Design review of the part built by this model. Coordinates are the model's own, in mm. A direction names the side the tool comes from. Round coordinates to 2 decimals unless told otherwise and drop trailing zeros. Write each loop counter-clockwise with the first axis right and the second up, starting at its lowest first coordinate (ties: lowest second). Pieces come first, ordered by that corner, then holes. Notation, with made-up numbers: (17, -27.5) -> (74, -27.5) arc R13 cw to (74, -7.5) -> close; hole circle Ø6 at (5.5, 6.25). An arc over 180 degrees is marked (long way). Write item = value, one per line. Start each with the question number.
Item 1: Add section D-D, the plane z = 12. State the section outline as (x, y) points, then the cut area to 3 significant figures.
Item 2: Machinability: for faces 1 (the cylindrical face through (20.8, 31.08, -2.11)), 2 (the cylindrical face through (12, 33, 0)), which of the approach directions +Z, -Z, +X, -X, +Y, -Y give a long, thin tool a straight path to every point of the face, cutting with its end or side? Answer none if there is none.
Item 3: Add section B-B, the plane x = 8. State the section outline as (y, z) points, then the cut area to 3 significant figures.
Item 4: To check wall thickness, follow L1, parallel to X at y = 0, z = -17.5; L2, parallel to X at y = 0, z = -16; L3, parallel to Y at x = 1.5, z = -0.5. State the ranges of each line that lie inside material, in increasing order.
Item 5: For pin 1 Ø23.5 at (y, z) = (0, 0) entering from +X; pin 2 Ø8.5 at (y, z) = (26, 0) entering from +X; pin 3 Ø5.5 at (y, z) = (25, 0.5) entering from +X; pin 4 Ø12 at (x, z) = (13.5, -1.5) entering from +Y, all flat-tipped, find the tip position at first contact; note any pin that passes through.
Item 6: Add section A-A, the plane y = 0. State the section outline as (x, z) points.
Item 7: Add section C-C, the plane x = 19.75. State the section outline as (y, z) points, then the cut area to 3 significant figures.
Item 8: Mouldability with a two-part tool opening along Z and no side actions: class faces 3 (the flat face through (24, -8, 15)), 4 (the cylindrical face through (8.86, 23.36, -2.02)), 5 (the cylindrical face through (12, -33, 0)) as released by +Z, released by -Z, zero draft, split by the parting line, or undercut.
Autodesk Inventor part; units mm, degrees
ref_plane "to_bearings_XY" through (16, 0, 0) normal (1, 0, 0) x (0, 0, -1)
ref_plane "to_bearings_YZ" through (16, 0, 0) normal (0, 0, -1) x (0, 1, 0)
ref_plane "to_bearings_ZX" through (16, 0, 0) normal (0, 1, 0) x (1, 0, 0)
sketch "Sketch_1" plane through (0, 0, 0) normal (0, 0, 1) x (1, 0, 0)
  line L0 (24, 0) -> (0, 0)
  line L1 (0, 33) -> (0, 13)
  line L2 (0, 13) -> (16, 13)
  line L3 (16, 13) -> (16, 16.5)
  line L4 (16, 16.5) -> (24, 16.5)
  line L5 (24, 16.5) -> (24, 33)
  line L6 (24, 33) -> (0, 33)
revolve "Revolution1" add sketch "Sketch_1" angle 360 about axis through (24, 0, 0) along (1, 0, 0)
sketch "Sketch_2" plane through (0, 0, 0) normal (1, 0, 0) x (0, 1, 0)
  line L0 (-132, 88) -> (-132, -88)
  line L1 (-132, -88) -> (132, -88)
  line L2 (132, -88) -> (132, 88)
  line L3 (132, 88) -> (-132, 88)
  line L4 (-33, 22) -> (-33, -22)
  line L5 (-33, -22) -> (33, -22)
  line L6 (33, -22) -> (33, 22)
  line L7 (33, 22) -> (-33, 22)
extrude "Extrusion1" cut sketch "Sketch_2" along normal blind 26
sketch "Sketch_3" plane through (0, 0, 0) normal (0, 0, 1) x (1, 0, 0)
  line L0 (24, 26) -> (0, 26)
  line L1 (0, 26) -> (0, 30)
  line L2 (0, 30) -> (0.6765, 29.3235)
  line L3 (0.6765, 29.3235) -> (16.8235, 29.3235)
  line L4 (16.8235, 29.3235) -> (17.5, 30)
  line L5 (17.5, 30) -> (17.5, 31.5)
  line L6 (17.5, 31.5) -> (24, 31.5)
  line L7 (24, 31.5) -> (24, 26)
  line L8 (24, 26) -> (0, 26)
revolve "Revolution2" cut sketch "Sketch_3" angle 360 about axis through (24, 26, 0) along (1, 0, 0)
thread "Thread1"
pattern_linear "Rectangular Pattern1" count 2 spacing 52 along (0, -1, 0) of "Revolution2"
sketch "Sketch_4" plane through (8, 0, 0) normal (1, 0, 0) x (0, 0, -1)
  line L0 (-12.65, 0) -> (-22, 0)
  line L1 (-22, 0) -> (-22, 2.5)
  line L2 (-22, 2.5) -> (-21.567, 2.067)
  line L3 (-21.567, 2.067) -> (-13.083, 2.067)
  line L4 (-13.083, 2.067) -> (-12.65, 2.5)
  line L5 (-12.65, 2.5) -> (-12.65, 0)
  line L6 (-12.65, 0) -> (-22, 0)
revolve "Revolution3" cut sketch "Sketch_4" angle 360 about axis through (8, 0, 12.65) along (0, 0, -1)
thread "Thread2"
sketch "Sketch_6" plane through (8, 0, 0) normal (1, 0, 0) x (0, 0, -1)
  line L0 (22, 0) -> (12.65, 0)
  line L1 (12.65, 0) -> (12.65, 2.5)
  line L2 (12.65, 2.5) -> (13.083, 2.067)
  line L3 (13.083, 2.067) -> (21.567, 2.067)
  line L4 (21.567, 2.067) -> (22, 2.5)
  line L5 (22, 2.5) -> (22, 0)
  line L6 (22, 0) -> (12.65, 0)
revolve "Revolution4" cut sketch "Sketch_6" angle 360 about axis through (8, 0, -22) along (0, 0, -1)
thread "Thread3"
ref_plane "to_bearings_XY" through (16, 0, 0) normal (1, 0, 0) x (0, 0, -1)
ref_plane "to_bearings_YZ" through (16, 0, 0) normal (0, 0, -1) x (0, 1, 0)
ref_plane "to_bearings_ZX" through (16, 0, 0) normal (0, 1, 0) x (1, 0, 0)
ref_plane "to_screw1_XY" through (8, 0, 13) normal (0, 0, 1) x (1, 0, 0)
ref_plane "to_screw1_YZ" through (8, 0, 13) normal (1, 0, 0) x (0, 1, 0)
ref_plane "to_screw1_ZX" through (8, 0, 13) normal (0, 1, 0) x (0, 0, 1)
ref_plane "to_screw2_XY" through (8, 0, -13) normal (0, 0, -1) x (1, 0, 0)
ref_plane "to_screw2_YZ" through (8, 0, -13) normal (1, 0, 0) x (0, -1, 0)
ref_plane "to_screw2_ZX" through (8, 0, -13) normal (0, -1, 0) x (0, 0, -1)
properties part number "BGCSB14_h"
Result set:
q1.outline = (0, -30.74) -> (24, -30.74) -> (24, -11.32) -> (16, -11.32) -> (16, -5) -> (0, -5) -> close; (0, 5) -> (16, 5) -> (16, 11.32) -> (24, 11.32) -> (24, 30.74) -> (0, 30.74) -> close
q1.area = 1,130 mm²
q2.face_1 = +X
q2.face_2 = +X, -X, +Y
q3.outline = (-24.6, -22) -> (-2.5, -22) -> (-2.07, -21.57) -> (-2.07, -13.08) -> (-2.37, -12.78) arc R13 cw to (-2.37, 12.78) -> (-2.07, 13.08) -> (-2.07, 21.57) -> (-2.5, 22) -> (-24.6, 22) arc R33 ccw to start; (2.07, -21.57) -> (2.5, -22) -> (24.6, -22) arc R33 ccw to (24.6, 22) -> (2.5, 22) -> (2.07, 21.57) -> (2.07, 13.08) -> (2.37, 12.78) arc R13 cw to (2.37, -12.78) -> (2.07, -13.08) -> close; hole circle Ø6.65 at (-26, 0); hole circle Ø6.65 at (26, 0)
q3.area = 2,000 mm²
q4.L1 = 0 to 5.93, 10.07 to 24
q4.L2 = 0 to 5.93, 10.07 to 16
q4.L3 = -33 to -29.29, -22.71 to -12.99, 12.99 to 22.71, 29.29 to 33
q5.pin_1 = through
q5.pin_2 = 17.5
q5.pin_3 = 17.37
q5.pin_4 = 33
q6.outline = (0, -22) -> (5.5, -22) -> (5.93, -21.57) -> (5.93, -13.08) -> (5.85, -13) -> (0, -13) -> close; (0, 13) -> (5.85, 13) -> (5.93, 13.08) -> (5.93, 21.57) -> (5.5, 22) -> (0, 22) -> close; (10.07, -21.57) -> (10.5, -22) -> (24, -22) -> (24, -16.5) -> (16, -16.5) -> (16, -13) -> (10.15, -13) -> (10.07, -13.08) -> close; (10.07, 13.08) -> (10.15, 13) -> (16, 13) -> (16, 16.5) -> (24, 16.5) -> (24, 22) -> (10.5, 22) -> (10.07, 21.57) -> close
q7.outline = (-24.6, -22) -> (24.6, -22) arc R33 ccw to (24.6, 22) -> (-24.6, 22) arc R33 ccw to start; hole circle Ø11 at (-26, 0); hole circle Ø33 at (0, 0); hole circle Ø11 at (26, 0)
q7.area = 1,630 mm²
q8.face_3 = zero draft
q8.face_4 = undercut
q8.face_5 = split by the parting line
